Answer from the drawing. Dimensions are ordinates in mm from the lowest x, y and z of the part. Coordinates: 2 decimals unless noted, no trailing zeros. Write each loop counter-clockwise with the first axis right and the second up, starting at its lowest first coordinate (ties: lowest second). Pieces come first, ordered by that corner, then holes. Notation, with made-up numbers: (74, -6) -> (110, -6) arc R26 cw to (110, 21) -> close; hole circle Ø3 at (39, 54.25). An arc over 180 degrees is marked (long way). One line per item, written item: value. Start each with the question number.
1. For a pull along Z with two mould halves and no side action, classify the marked faces 1, 2 and 3 as pulls with the +Z half, pulls with the -Z half, needs draft (parallel to the pull), parting line crosses it, or undercut.
2. Find section B-B, the plane z = 41.3. Write down the section's boundary in (x, y).
3. Find section A-A, the plane x = 41.3. Write down the section's boundary in (y, z).
4. Given P1, Ø3, axis at x = 66.5, y = 3, coming from the +Z side; P2, Ø0.8, axis at x = 79, y = 10.5, coming from the +Z side; P3, Ø1.5, axis at x = 64.5, y = 11.5, coming from the -Z side (1 decimal), each flat-ended and moving along its own axis, determine where each tip first touches the part or whether it passes through.
5. Consider line 1 along Y through (x, z) = (17, 61.5); line 2 along X through (y, z) = (12.15, 76.8) (1 decimal); line 3 along X through (y, z) = (8.25, 48.5). Determine where each line is inside the solid, lowest interval first.
6. Find section C-C, the plane y = 5.75. Write down the section's boundary in (x, z).
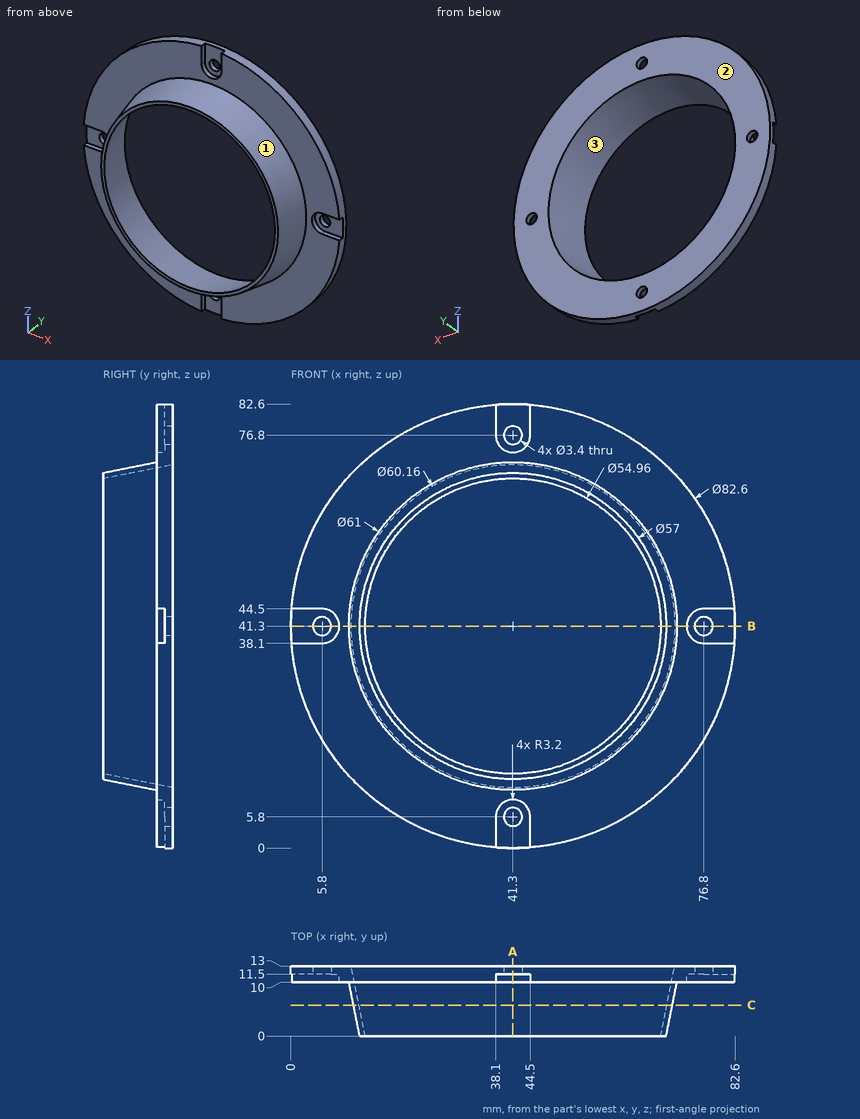
Answer block:
1. face 1: parting line crosses it
1. face 2: needs draft
1. face 3: undercut
2. outline: (0, 11.5) -> (4.1, 11.5) -> (4.1, 13) -> (0, 13) -> close; (7.5, 11.5) -> (9, 11.5) -> (9, 10) -> (10.8, 10) -> (12.8, 0) -> (13.82, 0) -> (11.22, 13) -> (7.5, 13) -> close; (68.78, 0) -> (69.8, 0) -> (71.8, 10) -> (73.6, 10) -> (73.6, 11.5) -> (75.1, 11.5) -> (75.1, 13) -> (71.38, 13) -> close; (78.5, 11.5) -> (82.6, 11.5) -> (82.6, 13) -> (78.5, 13) -> close
3. outline: (0, 12.8) -> (10, 10.8) -> (10, 9) -> (11.5, 9) -> (11.5, 7.5) -> (13, 7.5) -> (13, 11.22) -> (0, 13.82) -> close; (0, 68.78) -> (13, 71.38) -> (13, 75.1) -> (11.5, 75.1) -> (11.5, 73.6) -> (10, 73.6) -> (10, 71.8) -> (0, 69.8) -> close; (11.5, 0) -> (13, 0) -> (13, 4.1) -> (11.5, 4.1) -> close; (11.5, 78.5) -> (13, 78.5) -> (13, 82.6) -> (11.5, 82.6) -> close
4. P1: stops at z = 58.25
4. P2: stops at z = 59.03
4. P3: stops at z = 6.6
5. line 1: y = 10 to 13
5. line 2: x = 20.2 to 39.6, 43 to 62.4
5. line 3: x = 12.02 to 13.07, 69.53 to 70.58
6. outline: circle Ø59.3 at (41.3, 41.3); hole circle Ø57.26 at (41.3, 41.3)
